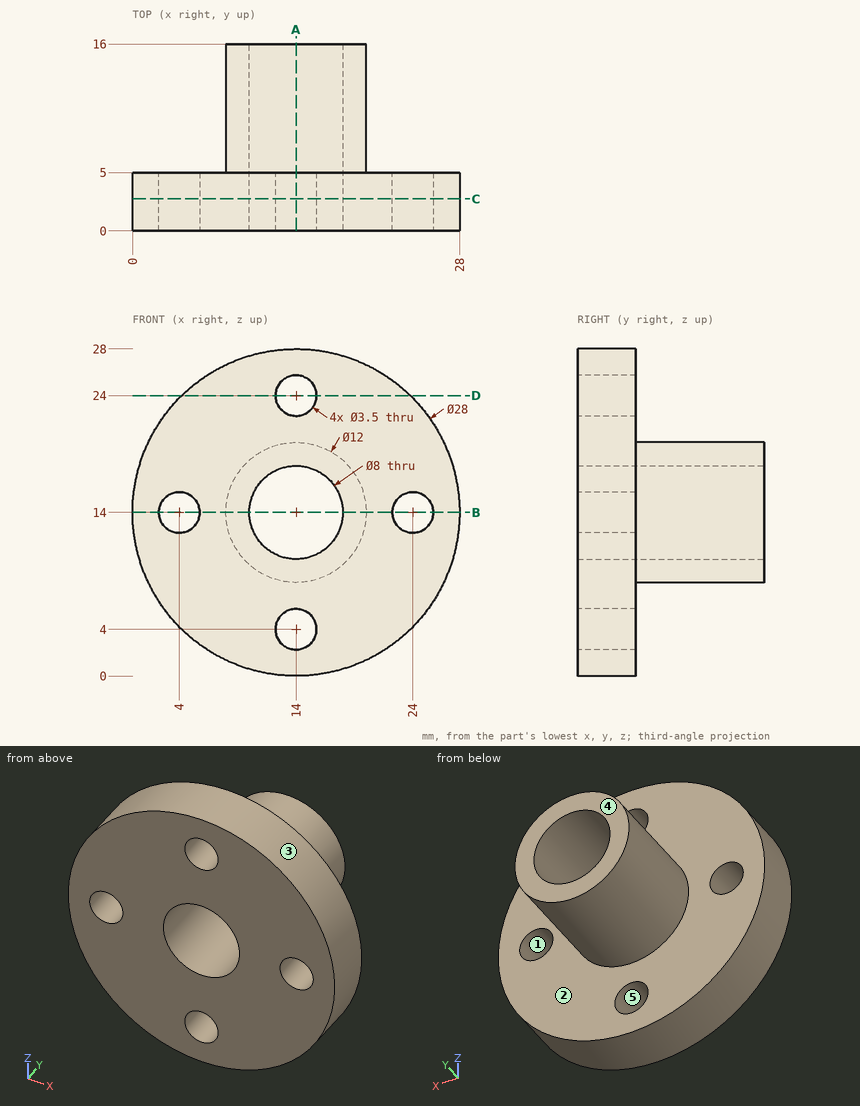
Here's the drawing with two shaded views (mm, measured from the low corner). I have some questions. A direction names the side the tool comes from. Give positions to 0.01 mm unless a question says otherwise; leave off trailing zeros. Loops run counter-clockwise (first coordinate to the right, second up) from the corner with the lowest first, then second, coordinate; pieces in that order, holes last. Notation, with made-up numbers: (25.5, 36) -> (41.5, 36) arc R28 cw to (41.5, 55) -> close; hole circle Ø4 at (-8, 80.25). An arc over 180 degrees is marked (long way). One line per item, written item: value.
Q1. I'm going to push flat-ended pins straight in: pin 1 Ø4 at (y, z) = (11.5, 8.5) entering from -X; pin 2 Ø2 at (y, z) = (1.5, 17) entering from -X; pin 3 Ø7 at (x, z) = (14, 14) entering from +Y; pin 4 Ø1 at (x, y) = (19.5, 9) entering from -Z. Where does each tip first touch, or does it pass through?
Answers follow:
pin 1: x = 9.13
pin 2: x = 0.14
pin 3: through
pin 4: z = 10.68
Q2. On a 3-axis mill with a long thin cutter (end or side, diameter ignored), from which of +Z, -Z, +X, -X, +Y, -Y can I reach the whole of each face in a straight line? I mean the marked faces 1 and 2. Say none if no direction works.
Answers follow:
face 1: +Y, -Y
face 2: +Y
Q3. Suppose I cut it at B-B on z = 14. Please give me the cut outline in (x, y).
Answers follow:
outline: (0, 0) -> (2.25, 0) -> (2.25, 5) -> (0, 5) -> close; (5.75, 0) -> (10, 0) -> (10, 16) -> (8, 16) -> (8, 5) -> (5.75, 5) -> close; (18, 0) -> (22.25, 0) -> (22.25, 5) -> (20, 5) -> (20, 16) -> (18, 16) -> close; (25.75, 0) -> (28, 0) -> (28, 5) -> (25.75, 5) -> close
Q4. If I drill on line 1 along Z through (x, y) = (14, 2.65); line 2 along Z through (x, y) = (14, 9.75); line 3 along Y through (x, z) = (6.25, 22), over which ranges is the centre line in solid material (lowest first)?
Answers follow:
line 1: 0 to 2.25, 5.75 to 10, 18 to 22.25, 25.75 to 28
line 2: 8 to 10, 18 to 20
line 3: 0 to 5
Q5. Suppose I cut it at D-D on z = 24. Please give me the cut outline in (x, y), then the cut area to 3 significant figures.
Answers follow:
outline: (4.2, 0) -> (12.25, 0) -> (12.25, 5) -> (4.2, 5) -> close; (15.75, 0) -> (23.8, 0) -> (23.8, 5) -> (15.75, 5) -> close
area: 80.5 mm^2
Q6. We'd pull the mould along X, two halves only. Please class the marked faces 3, 4 and 5: pulls with the +X half, pulls with the -X half, needs draft (parallel to the pull), parting line crosses it, or undercut.
Answers follow:
face 3: parting line crosses it
face 4: needs draft
face 5: undercut
Q7. Suppose I cut it at A-A on x = 14. Please give me the cut outline in (y, z), then the cut area to 3 significant figures.
Answers follow:
outline: (0, 0) -> (5, 0) -> (5, 2.25) -> (0, 2.25) -> close; (0, 5.75) -> (5, 5.75) -> (5, 8) -> (16, 8) -> (16, 10) -> (0, 10) -> close; (0, 18) -> (16, 18) -> (16, 20) -> (5, 20) -> (5, 22.25) -> (0, 22.25) -> close; (0, 25.75) -> (5, 25.75) -> (5, 28) -> (0, 28) -> close
area: 109 mm^2
Q8. Suppose I cut it at C-C on y = 2.75. Please give me the cut outline in (x, z), then the cut area to 3 significant figures.
Answers follow:
outline: circle Ø28 at (14, 14); hole circle Ø3.5 at (4, 14); hole circle Ø8 at (14, 14); hole circle Ø3.5 at (14, 4); hole circle Ø3.5 at (14, 24); hole circle Ø3.5 at (24, 14)
area: 527 mm^2
